Check sheet for the modelled part. Datum: model origin and axes. Units: mm. Face numbers are marked on the shaded views. A direction names the side the tool comes from. Round coordinates to 2 decimals unless told otherwise and drop trailing zeros. Order: outer loops, then holes, each group sorted by start corner. A loop starts at its lowest first (then second) coordinate and runs counter-clockwise, first axis right, second up. Notation, with made-up numbers: (75, 79.25) -> (114, 79.25) arc R19 ccw to (114, 107.25) -> close; hole circle Ø7 at (88, -39). An arc over 180 degrees is marked (long way). Use CSV: the item, a comma, the result in double quotes.
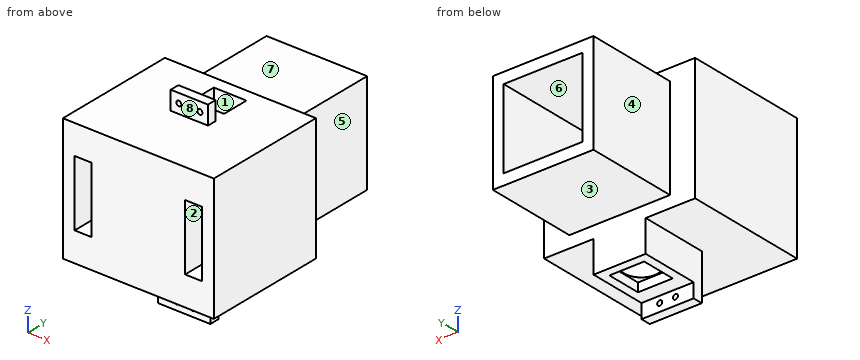
```python
from build123d import *

# Parameters (mm, degrees)
SKETCH_1_W          = 16.2
SKETCH_1_H          = 16.2
SKETCH_1_W_2        = 12.7
SKETCH_1_H_2        = 12.7
EXTRUDE_1_DEPTH     = 35
SKETCH_3_W          = 12.7
SKETCH_3_H          = 12.7
EXTRUDE_2_DEPTH     = 1
SKETCH_5_W          = 24.32
SKETCH_5_H          = 20
SKETCH_5_W_2        = 2.6
SKETCH_5_H_2        = 10.16
SKETCH_5_W_3        = 14.7
SKETCH_5_H_3        = 14.7
EXTRUDE_3_DEPTH     = 20
SKETCH_9_W          = 2.74
SKETCH_9_H          = 10.6
CUT_EXTRUDE_5_DEPTH = 8.7
CUT_EXTRUDE_6_REACH = 44.105
SKETCH_10_W         = 5.26
SKETCH_10_H         = 4.4
SKETCH_11_W         = 6
SKETCH_11_H         = 3
SKETCH_11_R         = 0.4
EXTRUDE_5_DEPTH     = 1.5
SKETCH_13_W         = 8.4
SKETCH_13_H         = 8.4
SKETCH_13_W_2       = 5.6
SKETCH_13_H_2       = 5.6
EXTRUDE_6_DEPTH     = 5.1
CUT_EXTRUDE_7_REACH = 45.61
SKETCH_15_R         = 2.65
SKETCH_16_W         = 8.4
SKETCH_16_H         = 1.6
EXTRUDE_7_DEPTH     = 7.4
CUT_EXTRUDE_8_REACH = 34.342
SKETCH_17_R         = 0.4
EXTRUDE_START       = 3.7
SKETCH_20_W         = 5.6
SKETCH_20_H         = 5.6
SKETCH_20_R         = 2.65
EXTRUDE_8_DEPTH     = 3.7
SKETCH_21_W         = 8.4
SKETCH_21_H         = 1
EXTRUDE_9_DEPTH     = 5.1


with BuildPart() as part:
    # Sketch 1 → Extrude 1 (new body)
    with BuildSketch(Plane(origin=(0, 0, 0), x_dir=(1, 0, 0), z_dir=(0, 1, 0))):
        Rectangle(SKETCH_1_W, SKETCH_1_H)
        Rectangle(SKETCH_1_W_2, SKETCH_1_H_2, mode=Mode.SUBTRACT)
    extrude(amount=EXTRUDE_1_DEPTH)



with BuildPart() as body_2:
    # Sketch 3 → Extrude 2 (new body)
    with BuildSketch(Plane(origin=(0, 0, 0), x_dir=(1, 0, 0), z_dir=(0, 1, 0))):
        Rectangle(SKETCH_3_W, SKETCH_3_H)
    extrude(amount=EXTRUDE_2_DEPTH)


with BuildPart() as part_1:
    add(part.part)

    add(body_2.part)  # Extrude 3 merges body 2
    # Sketch 5 → Extrude 3 (add)
    # profile 1 of 3: a face of its own
    with BuildSketch(Plane(origin=(0, 0, 0), x_dir=(1, 0, 0), z_dir=(0, 1, 0))):
        Rectangle(SKETCH_5_W, SKETCH_5_H)
        with Locations((-9.16, 0)):
            Rectangle(SKETCH_5_W_2, SKETCH_5_H_2, mode=Mode.SUBTRACT)
        Rectangle(SKETCH_5_W_3, SKETCH_5_H_3, mode=Mode.SUBTRACT)
        with Locations((9.16, 0)):
            Rectangle(SKETCH_5_W_2, SKETCH_5_H_2, mode=Mode.SUBTRACT)
    # profile 2 of 3: a face of its own
    with BuildSketch(Plane(origin=(0, 0, 0), x_dir=(1, 0, 0), z_dir=(0, 1, 0))):
        with Locations((-9.16, 0)):
            Rectangle(SKETCH_5_W_2, SKETCH_5_H_2)
    # profile 3 of 3: a face of its own
    with BuildSketch(Plane(origin=(0, 0, 0), x_dir=(1, 0, 0), z_dir=(0, 1, 0))):
        with Locations((9.16, 0)):
            Rectangle(SKETCH_5_W_2, SKETCH_5_H_2)
    extrude(amount=EXTRUDE_3_DEPTH)

    # Sketch 9 → Cut-Extrude 5 (cut)
    with BuildSketch(Plane(origin=(0, 0, 0), x_dir=(1, 0, 0), z_dir=(0, 1, 0))):
        with Locations((-8.89, 0)):
            Rectangle(SKETCH_9_W, SKETCH_9_H)
        with Locations((8.89, 0)):
            Rectangle(SKETCH_9_W, SKETCH_9_H)
    extrude(amount=CUT_EXTRUDE_5_DEPTH, mode=Mode.SUBTRACT)

    # Sketch 10 → Cut-Extrude 6 (cut, up to next)
    with BuildSketch(Plane.XY.offset(10), mode=Mode.PRIVATE) as cut_extrude_6_sk1:
        with Locations((0, 15.8)):
            Rectangle(SKETCH_10_W, SKETCH_10_H)
    cut_extrude_6_tool1 = extrude(cut_extrude_6_sk1.sketch, amount=-CUT_EXTRUDE_6_REACH, mode=Mode.PRIVATE) & part_1.part
    add(cut_extrude_6_tool1.solids().sort_by_distance((0, 15.8, 10))[0], mode=Mode.SUBTRACT)

    # Sketch 11 → Extrude 5 (add)
    with BuildSketch(Plane(origin=(0, 10, 0), x_dir=(1, 0, 0), z_dir=(0, 1, 0))):
        with Locations((0, -11.5)):
            Rectangle(SKETCH_11_W, SKETCH_11_H)
        with Locations(Location((-1.7, -11.5, 0), (0, 0, 270))):
            Circle(SKETCH_11_R, mode=Mode.SUBTRACT)
        with Locations(Location((1.7, -11.5, 0), (0, 0, 270))):
            Circle(SKETCH_11_R, mode=Mode.SUBTRACT)
    extrude(amount=EXTRUDE_5_DEPTH)

    # Sketch 13 → Extrude 6 (add)
    with BuildSketch(Plane(origin=(0, 0, -10), x_dir=(-1, 0, 0), z_dir=(0, 0, -1))):
        with Locations((0, 15.8)):
            Rectangle(SKETCH_13_W, SKETCH_13_H)
        with Locations((0, 15.8)):
            Rectangle(SKETCH_13_W_2, SKETCH_13_H_2, mode=Mode.SUBTRACT)
    extrude(amount=EXTRUDE_6_DEPTH)

    # Sketch 15 → Cut-Extrude 7 (cut, up to next)
    with BuildSketch(Plane(origin=(0, 0, -10), x_dir=(-1, 0, 0), z_dir=(0, 0, -1)), mode=Mode.PRIVATE) as cut_extrude_7_sk1:
        with Locations((0, 15.8)):
            Circle(SKETCH_15_R)
    cut_extrude_7_tool1 = extrude(cut_extrude_7_sk1.sketch, amount=-CUT_EXTRUDE_7_REACH, mode=Mode.PRIVATE) & part_1.part
    add(cut_extrude_7_tool1.solids().sort_by_distance((0, 15.8, -10))[0], mode=Mode.SUBTRACT)

    # Sketch 16 → Extrude 7 (add)
    with BuildSketch(Plane(origin=(0, 0, -10), x_dir=(-1, 0, 0), z_dir=(0, 0, -1))):
        with Locations((0, 9.8)):
            Rectangle(SKETCH_16_W, SKETCH_16_H)
    extrude(amount=EXTRUDE_7_DEPTH)

    # Sketch 17 → Cut-Extrude 8 (cut, up to next)
    with BuildSketch(Plane(origin=(0, 10.6, 0), x_dir=(1, 0, 0), z_dir=(0, 1, 0)), mode=Mode.PRIVATE) as cut_extrude_8_sk1:
        with Locations(Location((1.27, 16.15, 0), (0, 0, 270))):
            Circle(SKETCH_17_R)
    cut_extrude_8_tool1 = extrude(cut_extrude_8_sk1.sketch, amount=-CUT_EXTRUDE_8_REACH, mode=Mode.PRIVATE) & part_1.part
    # Sketch 17 → Cut-Extrude 8 (cut, up to next)
    with BuildSketch(Plane(origin=(0, 10.6, 0), x_dir=(1, 0, 0), z_dir=(0, 1, 0)), mode=Mode.PRIVATE) as cut_extrude_8_sk2:
        with Locations(Location((-1.27, 16.15, 0), (0, 0, 270))):
            Circle(SKETCH_17_R)
    cut_extrude_8_tool2 = extrude(cut_extrude_8_sk2.sketch, amount=-CUT_EXTRUDE_8_REACH, mode=Mode.PRIVATE) & part_1.part
    add(cut_extrude_8_tool1.solids().sort_by_distance((1.27, 10.6, -16.15))[0], mode=Mode.SUBTRACT)
    add(cut_extrude_8_tool2.solids().sort_by_distance((-1.27, 10.6, -16.15))[0], mode=Mode.SUBTRACT)

    # Sketch 20 → Extrude 8 (add)
    with BuildSketch(Plane(origin=(0, 0, -10), x_dir=(-1, 0, 0), z_dir=(0, 0, -1)).offset(EXTRUDE_START)):
        with Locations((0, 15.8)):
            Rectangle(SKETCH_20_W, SKETCH_20_H)
        with Locations((0, 15.8)):
            Circle(SKETCH_20_R, mode=Mode.SUBTRACT)
    extrude(amount=-EXTRUDE_8_DEPTH)

    # Sketch 21 → Extrude 9 (add)
    with BuildSketch(Plane(origin=(0, 0, -10), x_dir=(-1, 0, 0), z_dir=(0, 0, -1))):
        with Locations((0, 11.1)):
            Rectangle(SKETCH_21_W, SKETCH_21_H)
    extrude(amount=EXTRUDE_9_DEPTH)


solid = part_1.part
```
Q1. Go/stop test with flat-tipped pins: pin 1 (1.1 mm diameter, centred on x = 2, z = -16.5, fed in from +Y); pin 2 (5 mm diameter, centred on y = 31, z = -4.5, fed in from +X); pin 3 (1.5 mm diameter, centred on y = 17, z = -14.5, fed in from +X); pin 4 (4 mm diameter, centred on x = 0, y = 15.8, fed in from +Z). Record where each tip stops, or that it passes through.
Result sheet:
pin 1,"stops at y = 10.6"
pin 2,"stops at x = 8.1"
pin 3,"stops at x = 4.2"
pin 4,"passes through"
Q2. Scan lines: L1, parallel to X at y = 10.4, z = 11.5; L2, parallel to X at y = 7, z = 0.5; L3, parallel to Z at x = 1.75, y = 29. Record each from-to range of solid material in increasing order.
Result sheet:
L1,"x = -3 to -2.1, -1.3 to 1.3, 2.1 to 3"
L2,"x = -12.16 to -10.26, -7.52 to -6.35, 6.35 to 7.52, 10.26 to 12.16"
L3,"z = -8.1 to -6.35, 6.35 to 8.1"
Q3. Access from +Z, -Z, +X, -X, +Y, -Y to the whole of each face (thin tool, end or side, straight path). Record for the marked faces 1, 2, 3, 4 and 5.
Result sheet:
face 1,"+Z"
face 2,"-Y"
face 3,"-Z, +X, -X, +Y"
face 4,"+Z, -Z, -X, +Y"
face 5,"+Z, -Z, +X, +Y"
Q4. Sectioned sample at C-C, the plane y = 7. Enter the section's corners in (x, z), then the cut area to 3 significant figures.
Result sheet:
outline,"(-12.16, -10) -> (12.16, -10) -> (12.16, 10) -> (-12.16, 10) -> close; hole (-10.26, -5.3) -> (-7.52, -5.3) -> (-7.52, 5.3) -> (-10.26, 5.3) -> close; hole (-6.35, -6.35) -> (6.35, -6.35) -> (6.35, 6.35) -> (-6.35, 6.35) -> close; hole (7.52, -5.3) -> (10.26, -5.3) -> (10.26, 5.3) -> (7.52, 5.3) -> close"
area,"267 mm^2"
Q5. Sectioned sample at B-B, the plane x = -9.25. Enter the section's corners in (y, z), then the cut area to 3 significant figures.
Result sheet:
outline,"(0, -10) -> (20, -10) -> (20, 10) -> (0, 10) -> (0, 5.3) -> (8.7, 5.3) -> (8.7, -5.3) -> (0, -5.3) -> close"
area,"308 mm^2"
Q6. Sectioned sample at A-A, the plane y = 15.8. Enter the section's corners in (x, z), then the cut area to 3 significant figures.
Result sheet:
outline,"(-12.16, -10) -> (-4.2, -10) -> (-4.2, -15.1) -> (-2.8, -15.1) -> (-2.8, -13.7) -> (-2.65, -13.7) -> (-2.65, -6.35) -> (-6.35, -6.35) -> (-6.35, 6.35) -> (-2.63, 6.35) -> (-2.63, 10) -> (-12.16, 10) -> close; (2.63, 6.35) -> (6.35, 6.35) -> (6.35, -6.35) -> (2.65, -6.35) -> (2.65, -13.7) -> (2.8, -13.7) -> (2.8, -15.1) -> (4.2, -15.1) -> (4.2, -10) -> (12.16, -10) -> (12.16, 10) -> (2.63, 10) -> close"
area,"302 mm^2"
Q7. Sectioned sample at D-D, the plane z = 2. Enter the section's corners in (x, y), then the cut area to 3 significant figures.
Result sheet:
outline,"(-12.16, 0) -> (-10.26, 0) -> (-10.26, 8.7) -> (-7.52, 8.7) -> (-7.52, 0) -> (7.52, 0) -> (7.52, 8.7) -> (10.26, 8.7) -> (10.26, 0) -> (12.16, 0) -> (12.16, 20) -> (8.1, 20) -> (8.1, 35) -> (6.35, 35) -> (6.35, 1) -> (-6.35, 1) -> (-6.35, 35) -> (-8.1, 35) -> (-8.1, 20) -> (-12.16, 20) -> close"
area,"250 mm^2"
Q8. Mould release check, pull along Z, two halves, no side actions. Record for the marked faces 6, 7 and 8: pulls with the +Z half, pulls with the -Z half, needs draft (parallel to the pull), parting line crosses it, or undercut.
Result sheet:
face 6,"undercut"
face 7,"pulls with the +Z half"
face 8,"needs draft"
